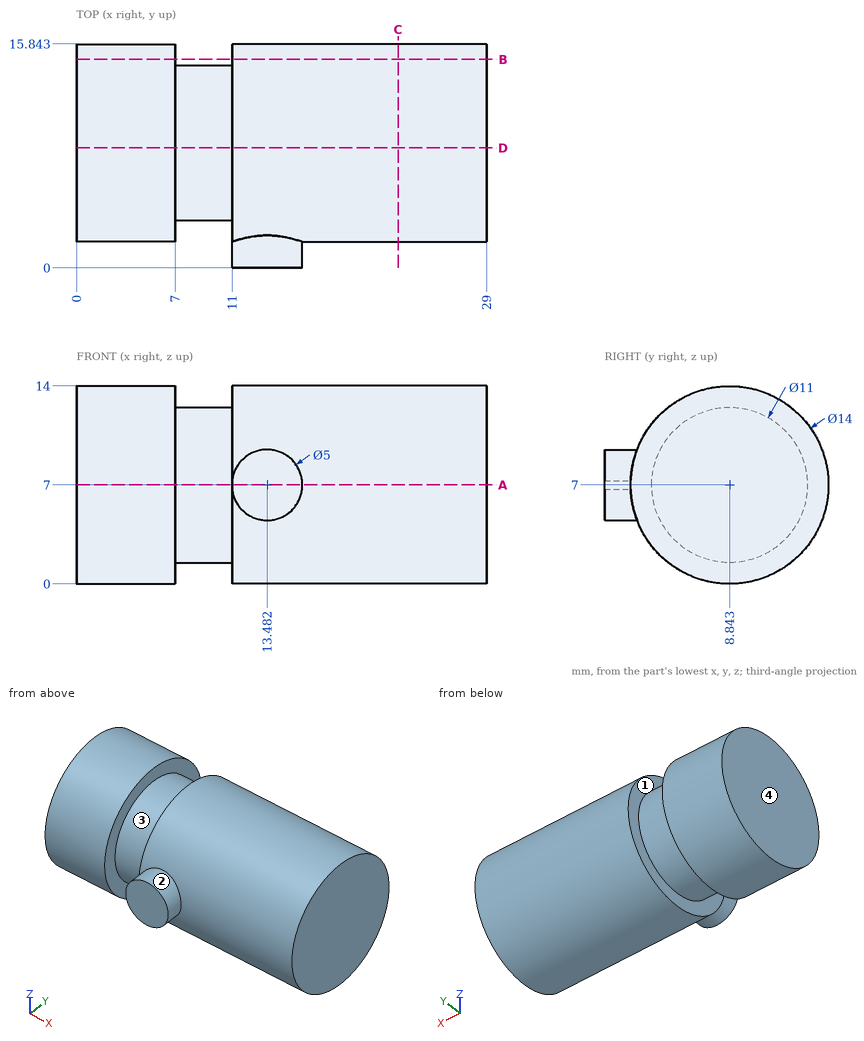
The figure shows three views and two pictorial views of one solid part (mm, origin at its lowest corner). Answer the questions. Round coordinates to 2 decimals unless told otherwise and drop trailing zeros. Order: outer loops, then holes, each group sorted by start corner. A loop starts at its lowest first (then second) coordinate and runs counter-clockwise, first axis right, second up.
Q1. A cutting plane is placed at B-B, the plane y = 14.75. Determine the outline of the cut face in (x, z), then the cut area to 3 significant figures.
Solution:
outline: (0, 3.24) - (7, 3.24) - (7, 10.76) - (0, 10.76) - close; (11, 3.24) - (29, 3.24) - (29, 10.76) - (11, 10.76) - close
area: 188 mm2
Q2. A cutting plane is placed at C-C, the plane x = 22.75. Determine the outline of the cut face in (y, z).
Solution:
outline: circle Ø14 at (8.84, 7)
Q3. The mould has two halves that part along X. Classify the marked faces 1, 2, 3 and 4: pulls with the +X half, pulls with the -X half, needs draft (parallel to the pull), parting line crosses it, or undercut.
Solution:
face 1: undercut
face 2: parting line crosses it
face 3: undercut
face 4: pulls with the -X half
Q4. A cutting plane is placed at D-D, the plane y = 8.5. Determine the outline of the cut face in (x, z).
Solution:
outline: (0, 0.01) - (7, 0.01) - (7, 1.51) - (11, 1.51) - (11, 0.01) - (29, 0.01) - (29, 13.99) - (11, 13.99) - (11, 12.49) - (7, 12.49) - (7, 13.99) - (0, 13.99) - close
Q5. Given pin 1 Ø1 at (x, y) = (23, 14) entering from -Z; pin 2 Ø1 at (y, z) = (3.5, 12.5) entering from +X; pin 3 Ø3 at (x, z) = (26, 12) entering from -Y; pin 4 Ø3 at (x, y) = (10, 12.5) entering from -Z, each flat-ended and moving along its own axis, determine where each tip first touches the part or whether it passes through.
Solution:
pin 1: stops at z = 1.77
pin 2: passes through
pin 3: stops at y = 2.78
pin 4: stops at z = 0.48
Q6. A cutting plane is placed at A-A, the plane z = 7. Determine the outline of the cut face in (x, y), then the cut area to 3 significant figures.
Solution:
outline: (0, 1.84) - (7, 1.84) - (7, 3.34) - (11, 3.34) - (11, 0) - (15.98, 0) - (15.98, 1.84) - (29, 1.84) - (29, 15.84) - (11, 15.84) - (11, 14.34) - (7, 14.34) - (7, 15.84) - (0, 15.84) - close
area: 403 mm2
Q7. Find the intervals of material crossed by line 1 along X through (y, z) = (11.5, 13.25); line 2 along Y through (x, z) = (22, 7.25); line 3 along Z through (x, y) = (5, 9), in increasing order.
Solution:
line 1: x = 0 to 7, 11 to 29
line 2: y = 1.85 to 15.84
line 3: z = 0 to 14
